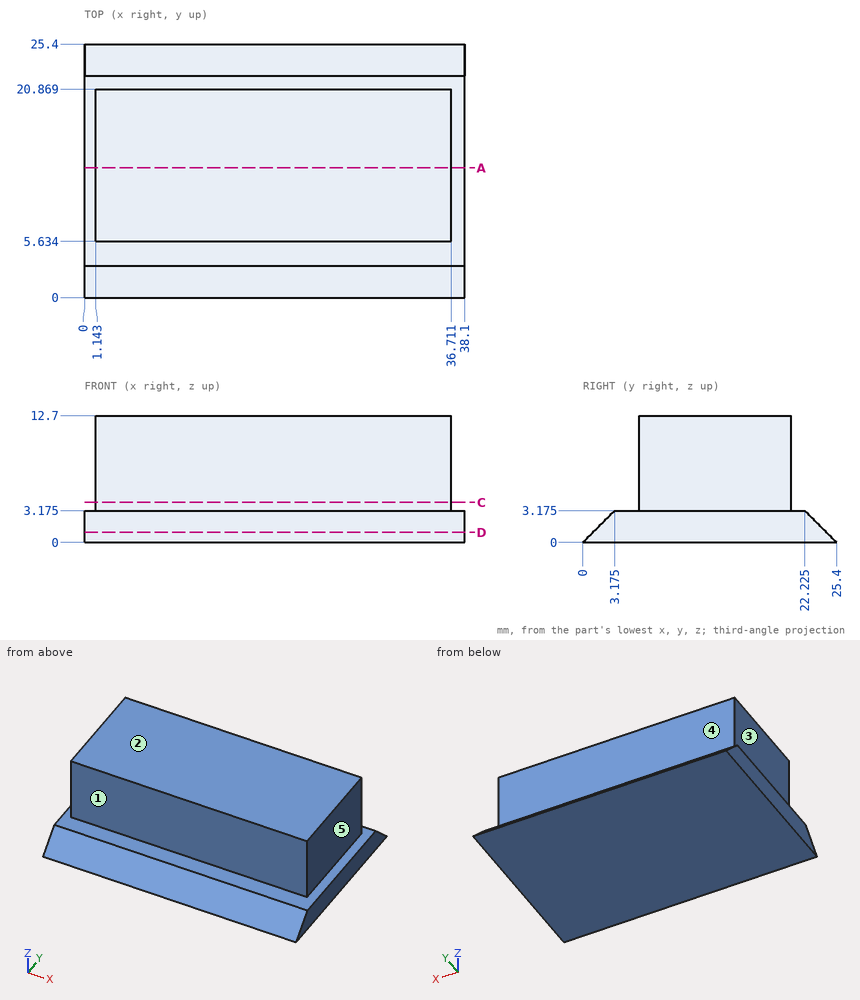
Source: three-view drawing plus pictorial views. Frame: mm from the lowest corner of the part. A direction names the side the tool comes from. Give positions to 0.01 mm unless a question says otherwise; leave off trailing zeros. Loops run counter-clockwise (first coordinate to the right, second up) from the corner with the lowest first, then second, coordinate; pieces in that order, holes last. Notation, with made-up numbers: (-12, -31.5) -> (45, -31.5) arc R27 ccw to (45, -11.5) -> close; hole circle Ø3 at (-5.5, -20). An arc over 180 degrees is marked (long way). Use a Markdown table: item, result. Add a question column.
(1) Access query for the marked faces 1, 2, 3, 4 and 5. Directions: +Z, -Z, +X, -X, +Y, -Y. A direction counts if a zero-diameter tool reaches every point of the face in a straight line with its end or side. Return the directions, or none.
(2) Ray query, line 1 (X direction, y = 20.5, z = 3.25); line 2 (Y direction, x = 23.5, z = 10); line 3 (Z direction, x = 9, y = 4.25) (1 decimal). Return the intervals inside material, ascending.
(3) Section query C-C (z = 4). Output: boundary loops of the cut face in (x, y).
(4) First-contact query: pin 1 Ø4 at (y, z) = (13.5, 10.5) entering from +X; pin 2 Ø5 at (y, z) = (14.5, 9.5) entering from -X; pin 3 Ø5 at (x, z) = (15, 9) entering from +Y. Flat tips, straight axial feed; report the tip coordinate or a pass-through.
(5) Section query D-D (z = 1). Output: boundary loops of the cut face in (x, y).
(6) Section query A-A (y = 13). Output: boundary loops of the cut face in (x, z) (1 decimal), then the cut area to 3 significant figures.
Checked values:
| question | item | result |
|---|---|---|
| 1 | face 1 | +Z, +X, -X, -Y |
| 1 | face 2 | +Z, +X, -X, +Y, -Y |
| 1 | face 3 | +Z, -X, +Y, -Y |
| 1 | face 4 | +Z, +X, -X, +Y |
| 1 | face 5 | +Z, +X, +Y, -Y |
| 2 | line 1 | 1.14 to 36.71 |
| 2 | line 2 | 5.63 to 20.87 |
| 2 | line 3 | 0 to 3.2 |
| 3 | outline | (1.14, 5.63) -> (36.71, 5.63) -> (36.71, 20.87) -> (1.14, 20.87) -> close |
| 4 | pin 1 | x = 36.71 |
| 4 | pin 2 | x = 1.14 |
| 4 | pin 3 | y = 20.87 |
| 5 | outline | (0, 1) -> (38.1, 1) -> (38.1, 24.4) -> (0, 24.4) -> close |
| 6 | outline | (0, 0) -> (38.1, 0) -> (38.1, 3.2) -> (36.7, 3.2) -> (36.7, 12.7) -> (1.1, 12.7) -> (1.1, 3.2) -> (0, 3.2) -> close |
| 6 | area | 460 mm^2 |
